Can you work these out from the model? Positions are in its coordinate system, mm. Give positions to 0.01 mm unless a question says otherwise; leave off trailing zeros. Order: outer loops, then holes, each group sorted by start corner. A loop starts at its lowest first (then second) coordinate and runs counter-clockwise, first axis right, second up. Notation, with made-up numbers: M -21,46 L 18,46 A32 ccw 18,77 Z; hole C 73,-15 d3. An arc over 180 degrees is marked long. Answer as a JSON object with one key per item and string values.
```python
from build123d import *

# Parameters (mm, degrees)
F0_W     = 195
F0_H     = 105
F0_R     = 5.5
F1_DEPTH = 18
F2_SIZE  = 0.5


with BuildPart() as f1:
    # F0 (on Front) → F1 (new body)
    with BuildSketch(Plane.XZ):
        Rectangle(F0_W, F0_H)
        with Locations((-80, -40)):
            Circle(F0_R, mode=Mode.SUBTRACT)
        with Locations((-20, -40)):
            Circle(F0_R, mode=Mode.SUBTRACT)
        with Locations((22.5, -40)):
            Circle(F0_R, mode=Mode.SUBTRACT)
        with Locations((82.5, -40)):
            Circle(F0_R, mode=Mode.SUBTRACT)
        with Locations((-80, 0)):
            Circle(F0_R, mode=Mode.SUBTRACT)
        with Locations((-20, 0)):
            Circle(F0_R, mode=Mode.SUBTRACT)
        with Locations((-80, 40)):
            Circle(F0_R, mode=Mode.SUBTRACT)
        with Locations((-20, 40)):
            Circle(F0_R, mode=Mode.SUBTRACT)
        with Locations((22.5, 0)):
            Circle(F0_R, mode=Mode.SUBTRACT)
        with Locations((82.5, 0)):
            Circle(F0_R, mode=Mode.SUBTRACT)
        with Locations((22.5, 40)):
            Circle(F0_R, mode=Mode.SUBTRACT)
        with Locations((82.5, 40)):
            Circle(F0_R, mode=Mode.SUBTRACT)
    extrude(amount=F1_DEPTH)

    # F2
    f2_edges = [f1.edges().sort_by_distance(p)[0] for p in [
        (-74.5, -9, 40),
        (-85.5, 0, 40),
        (-85.5, -18, 40),
        (-74.5, -9, 0),
        (-85.5, 0, 0),
        (-85.5, -18, 0),
        (-74.5, -9, -40),
        (-85.5, 0, -40),
        (-85.5, -18, -40),
        (-14.5, -9, 40),
        (-25.5, 0, 40),
        (-25.5, -18, 40),
        (-14.5, -9, 0),
        (-25.5, 0, 0),
        (-25.5, -18, 0),
        (-14.5, -9, -40),
        (-25.5, 0, -40),
        (-25.5, -18, -40),
        (28, -9, 40),
        (17, 0, 40),
        (17, -18, 40),
        (28, -9, 0),
        (17, 0, 0),
        (17, -18, 0),
        (28, -9, -40),
        (17, 0, -40),
        (17, -18, -40),
        (88, -9, 40),
        (77, 0, 40),
        (77, -18, 40),
        (88, -9, 0),
        (77, 0, 0),
        (77, -18, 0),
        (88, -9, -40),
        (77, 0, -40),
        (77, -18, -40),
    ]]
    chamfer(f2_edges, length=F2_SIZE)


solid = f1.part
```
1) I'm going to push a flat-ended pin straight in: pin 1 Ø9 at (x, z) = (-20, -40) entering from +Y. Where does the tip first touch, or does it pass through?
Results found:
{"pin 1": "passes through"}
2) I want a section at B-B on y = -4. Count the separate pieces of the cut face and the enclosed holes in it, and give its area (3 significant figures).
Results found:
{"separate pieces": "1", "enclosed holes": "12", "area": "19,300 mm²"}
3) I want a section at A-A on x = -80. Write out the boundary of the cut face in (y, z).
Results found:
{"outline": "M -18,-52.5 L 0,-52.5 L 0,-46 L -0.5,-45.5 L -17.5,-45.5 L -18,-46 Z; M -18,-34 L -17.5,-34.5 L -0.5,-34.5 L 0,-34 L 0,-6 L -0.5,-5.5 L -17.5,-5.5 L -18,-6 Z; M -18,6 L -17.5,5.5 L -0.5,5.5 L 0,6 L 0,34 L -0.5,34.5 L -17.5,34.5 L -18,34 Z; M -18,46 L -17.5,45.5 L -0.5,45.5 L 0,46 L 0,52.5 L -18,52.5 Z"}
4) I need wall thicknesses on L1, parallel to Z at x = -80, y = -11.25; L2, parallel to X at y = -2.75, z = -2; L3, parallel to Z at x = -77, y = -4. Which ranges of each line are inside material? Lowest first, please.
Results found:
{"L1": "z = -52.5 to -45.5, -34.5 to -5.5, 5.5 to 34.5, 45.5 to 52.5", "L2": "x = -97.5 to -85.12, -74.88 to -25.12, -14.88 to 17.38, 27.62 to 77.38, 87.62 to 97.5", "L3": "z = -52.5 to -44.61, -35.39 to -4.61, 4.61 to 35.39, 44.61 to 52.5"}
5) Thinking about a two-plate mould opening in Z: for faces 1 (the face through (21.784, -8.881, -34.547)), 2 (the face through (-97.5, -9, -1)), 3 (the face through (-1, -9, -52.5)), which applies, pulls with the +Z half, pulls with the -Z half, needs draft (parallel to the pull), parting line crosses it, or undercut?
Results found:
{"face 1": "undercut", "face 2": "needs draft", "face 3": "pulls with the -Z half"}
